Check sheet for the modelled part. Datum: model origin and axes. Units: mm. A direction names the side the tool comes from. Give positions to 0.01 mm unless a question says otherwise; leave off trailing zeros. Order: outer loops, then holes, each group sorted by start corner. A loop starts at its lowest first (then second) coordinate and runs counter-clockwise, first axis right, second up.
Item 1: Sectioned sample at C-C on y = 3.5. Count the separate pieces of the cut face and the enclosed holes in it, and give its area (3 significant figures).
Item 2: Sectioned sample at B-B on z = 144.5. Record the boundary of the cut face in (x, y).
Item 3: Material ranges on line 1 along Y through (x, z) = (8.5, 228); line 2 along X through (y, z) = (13.5, 15), recorded low to high.
Item 4: Release check for a two-part mould opening along X. For faces 3 (the flat face through (17.977, 10, 92)), 4 (the flat face through (3, -15.664, 118)), 5 (the flat face through (18.977, 10, 92)), 6 (the flat face through (3, 37.136, 118)) record: released by +X, released by -X, zero draft, split by the parting line, or undercut.
Item 5: Sectioned sample at D-D on z = 113. Record the boundary of the cut face in (x, y).
Item 6: Access from +Z, -Z, +X, -X, +Y, -Y to the whole of each face (thin tool, end or side, straight path). Record for faces 1 (the flat face through (-13.023, 10, 92)), 2 (the flat face through (-12.023, 10, 92)).
Item 7: Sectioned sample at A-A on x = 11.5. Record the boundary of the cut face in (y, z), and give its area (3 significant figures).
from build123d import *

# Parameters (mm, degrees)
ESQUISSE1_W                = 32
ESQUISSE1_H                = 53.8
ESQUISSE1_W_2              = 30
ESQUISSE1_H_2              = 51.8
BOSS_EXTRU_1_DEPTH         = 240
ESQUISSE2_W                = 5
ESQUISSE2_H                = 46.8
ENL_V_MAT_EXTRU_1_DEPTH    = 32
R_P_TITION_LIN_AIRE1_COUNT = 19
R_P_TITION_LIN_AIRE1_PITCH = 12.5


with BuildPart() as part:
    # Esquisse1 → Boss.-Extru.1 (new body)
    with BuildSketch(Plane.XY):
        with Locations((2.977116986, 10.236099585)):
            Rectangle(ESQUISSE1_W, ESQUISSE1_H)
        with Locations((2.977116986, 10.236099585)):
            Rectangle(ESQUISSE1_W_2, ESQUISSE1_H_2, mode=Mode.SUBTRACT)
    extrude(amount=BOSS_EXTRU_1_DEPTH)

    # Esquisse2 → Enlèv. mat.-Extru.1 (cut)
    with BuildSketch(Plane(origin=(18.977116986, 0, 0), x_dir=(0, 0, -1), z_dir=(1, 0, 0))):
        with Locations((-7.5, 8.736099585)):
            Rectangle(ESQUISSE2_W, ESQUISSE2_H)
    enl_v_mat_extru_1 = extrude(amount=-ENL_V_MAT_EXTRU_1_DEPTH, mode=Mode.SUBTRACT)

    # Répétition linéaire1: Enlèv. mat.-Extru.1 ×19
    with Locations(*[(0, 0, i * R_P_TITION_LIN_AIRE1_PITCH) for i in range(1, R_P_TITION_LIN_AIRE1_COUNT)]):
        add(enl_v_mat_extru_1, mode=Mode.SUBTRACT)


solid = part.part
Report:
1. separate pieces: 40
1. enclosed holes: 0
1. area: 290 mm2
2. outline: (-13.02, -16.66) - (18.98, -16.66) - (18.98, -14.66) - (17.98, -14.66) - (17.98, -15.66) - (-12.02, -15.66) - (-12.02, -14.66) - (-13.02, -14.66) - close; (-13.02, 32.14) - (-12.02, 32.14) - (-12.02, 36.14) - (17.98, 36.14) - (17.98, 32.14) - (18.98, 32.14) - (18.98, 37.14) - (-13.02, 37.14) - close
3. line 1: y = -16.66 to -15.66, 36.14 to 37.14
3. line 2: x = -13.02 to -12.02, 17.98 to 18.98
4. face 3: undercut
4. face 4: undercut
4. face 5: released by +X
4. face 6: zero draft
5. outline: (-13.02, -16.66) - (18.98, -16.66) - (18.98, 37.14) - (-13.02, 37.14) - close; hole (-12.02, -15.66) - (17.98, -15.66) - (17.98, 36.14) - (-12.02, 36.14) - close
6. face 1: +Z, -Z, -X, +Y, -Y
6. face 2: +Z, -Z
7. outline: (-16.66, 0) - (-15.66, 0) - (-15.66, 240) - (-16.66, 240) - close; (36.14, 0) - (37.14, 0) - (37.14, 240) - (36.14, 240) - close
7. area: 480 mm2
